```python
from build123d import *

# Parameters (mm, degrees)
F0_R     = 3
F1_DEPTH = 69.85
F5_DEPTH = 25
F6_DEPTH = 10.9
F8_DEPTH = 25
F9_DEPTH = 25


with BuildPart() as f1:
    # F0 (on Front) → F1 (new body)
    with BuildSketch(Plane.XZ):
        Circle(F0_R)
    extrude(amount=F1_DEPTH)

    # F2 (on Top) → F3 (revolve)
    with BuildSketch(Plane.XY):
        Polygon((-4.683842, 0), (0, 0), (0, 8.863604), align=None)
    revolve(axis=Axis((0, 4.431802, 0), (0, 1, 0)))

    # F4 (on Top) → F5 (cut)
    with BuildSketch(Plane.XY):
        Polygon((1.431932, 6.093189), (-1.507714, 6.047257), (-1.507714, -5.068278), (1.431932, -5.068278), align=None)
    extrude(amount=-F5_DEPTH, mode=Mode.SUBTRACT)

    # F4 (on Top) → F6 (cut)
    with BuildSketch(Plane.XY):
        Polygon((1.431932, 6.093189), (-1.507714, 6.047257), (-1.507714, -5.068278), (1.431932, -5.068278), align=None)
    extrude(amount=F6_DEPTH, mode=Mode.SUBTRACT)

    # F7 (on Top) → F8 (cut)
    with BuildSketch(Plane.XY):
        Polygon((0, 8.892538), (-1.547059, 5.977397), (1.504442, 6.018774), align=None)
    extrude(amount=-F8_DEPTH, mode=Mode.SUBTRACT)

    # F7 (on Top) → F9 (cut)
    with BuildSketch(Plane.XY):
        Polygon((0, 8.892538), (-1.547059, 5.977397), (1.504442, 6.018774), align=None)
    extrude(amount=F9_DEPTH, mode=Mode.SUBTRACT)


solid = f1.part
```
Read the model definition and answer for the solid it produces. Units are mm, in the model's axes. A direction names the side the tool comes from. Coordinates: 2 decimals unless noted, no trailing zeros. Order: outer loops, then holes, each group sorted by start corner. A loop starts at its lowest first (then second) coordinate and runs counter-clockwise, first axis right, second up. Notation, with made-up numbers: (70, 83.25) - (121, 83.25) arc R33 ccw to (121, 114.25) - close; hole circle Ø5 at (71.25, 38.25). An arc over 180 degrees is marked (long way). Answer as a JSON object with one key per item and string values. Group by question number.
Item 1: Section A-A (x = 0) is taken. Give the vertices of the cut face in (y, z).
Item 2: Section B-B (y = -15.5) is taken. Give the vertices of the cut face in (x, z).
Item 3: The mould has two halves that part along X. Classify faces 1 (the face through (0, -34, 3)), 2 (the face through (0, -69.85, 0)), 3 (the face through (-1.508, 1, 0)): +X half, -X half, draft (parallel to the pull), parting line (faces both ways), or undercut.
Item 4: Consider probe 1 along Y at (x, z) = (3, 0.75); probe 2 along Y at (x, z) = (1.25, 0); probe 3 along X at (y, z) = (-48.5, 0.5). Determine where each line is inside the solid, lowest interval first. Write a range as from..to.
Item 5: A tool of negligible diameter and unlimited length cuts with its end or side. For faces 4 (the face through (3.4, 0, 0.1)), 5 (the face through (-3.4, 0, 0.1)), 6 (the face through (-3.126, 2.947, -0.054)), 7 (the face through (3.115, 2.967, 0.055)), 8 (the face through (0, -5.068, 0)), from which of +Z, -Z, +X, -X, +Y, -Y can it reach the whole face along a straight path? Write none if from no direction.
Item 6: Flat-ended cylindrical pins translate along their axes: P1, Ø3, axis at x = 2.5, y = -30, coming from the -Z side; P2, Ø2, axis at x = 2.5, y = -16.5, coming from the +Z side; P3, Ø1.6, axis at x = 3, z = 1.5, coming from the -Y side; P4, Ø3, axis at x = -0.5, z = -2.5, coming from the +Y side. Find the tip coordinate at first contact, or state that the pin passes through.
Results are:
{
 "1": {"outline": "(-69.85, -3) - (-5.07, -3) - (-5.07, 3) - (-69.85, 3) - close"},
 "2": {"outline": "circle Ø6 at (0, 0)"},
 "3": {"face 1": "parting line", "face 2": "draft", "face 3": "undercut"},
 "4": {"probe 1": "y = 0..3.01", "probe 2": "y = -69.85..-5.07", "probe 3": "x = -2.96..2.96"},
 "5": {"face 4": "+X, -Y", "face 5": "-X, -Y", "face 6": "-X, +Y", "face 7": "+X, +Y", "face 8": "+Z, -Z, +Y"},
 "6": {"P1": "stops at z = -2.83", "P2": "stops at z = 2.6", "P3": "stops at y = -69.85", "P4": "stops at y = 4.98"}
}
